The listing builds one solid part. Answer for the finished solid, in the listing's coordinates (mm). A direction names the side the tool comes from. Round coordinates to 2 decimals unless told otherwise and drop trailing zeros. Loops run counter-clockwise (first coordinate to the right, second up) from the corner with the lowest first, then second, coordinate; pieces in that order, holes last. Notation, with made-up numbers: M -40,8 L 12,8 A31 ccw 12,40 Z; hole C -24,10 d10. An arc over 180 degrees is marked long. Put each result on its own line as item: value. Start each with the question number.
(1) Which of the six approach directions +Z, -Z, +X, -X, +Y, -Y give full straight-line access (tool end or side, diameter ignored) to faces 4 (the face through (-17.02, -29.06, -7.32)), 5 (the face through (-23, 0, 0)), 6 (the face through (11.923, 3.755, 15.226))?
(2) Determine the mould class of faces 1 (the face through (-17.86, 17.92, -0.15)), 2 (the face through (20.48, -23.343, 0.175)), 3 (the face through (0, 0, 16.5)) for opening direction Z: released by +Z, released by -Z, zero draft, split by the parting line, or undercut.
(3) Section A-A, the plane z = 9 is taken. Determine the outline of the cut face in (x, y), then the cut area to 3 significant figures.
(4) Section D-D, the plane z = -6.5 is taken. Count the separate pieces of the cut face and the enclosed holes in it, then the cut area to 3 significant figures.
(5) Section C-C, the plane y = -27 is taken. Determine the outline of the cut face in (x, z).
(6) Straight lines are drawn through the part: line 1 (Y direction, x = 21, z = -4.25); line 2 (Y direction, x = -9.5, z = 9). For each, find the intervals that lie inside material, in ascending order.
(7) Flat-ended cylindrical pins translate along their axes: P1, Ø3, axis at x = -21, y = -21, coming from the +Z side; P2, Ø22, axis at x = 2.5, y = -2, coming from the +Z side; P3, Ø10.5, axis at x = -4, z = 3, coming from the -Y side; P4, Ø13, axis at x = 0, y = 0, coming from the +Z side. Find the tip coordinate at first contact, or state that the pin passes through.
```python
from build123d import *

# Parameters (mm, degrees)
SKETCH1_W            = 50
SKETCH1_H            = 50
BOSS_EXTRUDE1_DEPTH  = 12.5
SKETCH2_R            = 12.5
BOSS_EXTRUDE2_DEPTH  = 5
CUT_EXTRUDE1_REACH   = 45.301
SKETCH4_R            = 2.4
SKETCH5_R            = 13
BOSS_EXTRUDE3_DEPTH  = 1
SHELL1_START         = -10.5
SHELL1_DEPTH         = 21
SHELL1_START_2       = 10.5
SHELL1_2_OUTLINE_R   = 10.5
SHELL1_2_DEPTH       = 4
SHELL1_3_OUTLINE_R   = 11
SHELL1_3_OUTLINE_R_2 = 10.5
SHELL1_3_DEPTH       = 1
FILLET1_R            = 3
SKETCH6_R            = 10
CUT_EXTRUDE2_DEPTH   = 1
FILLET2_R            = 1
CHAMFER1_SIZE        = 0.5
SKETCH7_R            = 2.5
BOSS_EXTRUDE4_DEPTH  = 8
BOSS_EXTRUDE4_TAPER  = 5


# Read off the part's stored shape, not the designer's step: Shell1
with BuildPart() as part:
    # Sketch1 → Boss-Extrude1 (new, symmetric)
    with BuildSketch(Plane.XY):
        Rectangle(SKETCH1_W, SKETCH1_H)
    extrude(amount=BOSS_EXTRUDE1_DEPTH, both=True)

    # Sketch2 → Boss-Extrude2 (add)
    with BuildSketch(Plane.XY.offset(12.5)):
        Circle(SKETCH2_R)
    extrude(amount=BOSS_EXTRUDE2_DEPTH)

    # Sketch4 → Cut-Extrude1 (cut, up to next)
    with BuildSketch(Plane.XY.offset(12.5), mode=Mode.PRIVATE) as cut_extrude1_sk1:
        with Locations((-21, 21)):
            Circle(SKETCH4_R)
    cut_extrude1_tool1 = extrude(cut_extrude1_sk1.sketch, amount=-CUT_EXTRUDE1_REACH, mode=Mode.PRIVATE) & part.part
    # Sketch4 → Cut-Extrude1 (cut, up to next)
    with BuildSketch(Plane.XY.offset(12.5), mode=Mode.PRIVATE) as cut_extrude1_sk2:
        with Locations((21, 21)):
            Circle(SKETCH4_R)
    cut_extrude1_tool2 = extrude(cut_extrude1_sk2.sketch, amount=-CUT_EXTRUDE1_REACH, mode=Mode.PRIVATE) & part.part
    # Sketch4 → Cut-Extrude1 (cut, up to next)
    with BuildSketch(Plane.XY.offset(12.5), mode=Mode.PRIVATE) as cut_extrude1_sk3:
        with Locations((-21, -21)):
            Circle(SKETCH4_R)
    cut_extrude1_tool3 = extrude(cut_extrude1_sk3.sketch, amount=-CUT_EXTRUDE1_REACH, mode=Mode.PRIVATE) & part.part
    # Sketch4 → Cut-Extrude1 (cut, up to next)
    with BuildSketch(Plane.XY.offset(12.5), mode=Mode.PRIVATE) as cut_extrude1_sk4:
        with Locations((21, -21)):
            Circle(SKETCH4_R)
    cut_extrude1_tool4 = extrude(cut_extrude1_sk4.sketch, amount=-CUT_EXTRUDE1_REACH, mode=Mode.PRIVATE) & part.part
    add(cut_extrude1_tool1.solids().sort_by_distance((-21, 21, 12.5))[0], mode=Mode.SUBTRACT)
    add(cut_extrude1_tool2.solids().sort_by_distance((21, 21, 12.5))[0], mode=Mode.SUBTRACT)
    add(cut_extrude1_tool3.solids().sort_by_distance((-21, -21, 12.5))[0], mode=Mode.SUBTRACT)
    add(cut_extrude1_tool4.solids().sort_by_distance((21, -21, 12.5))[0], mode=Mode.SUBTRACT)

    # Sketch5 → Boss-Extrude3 (add)
    with BuildSketch(Plane.XY.offset(12.5)):
        Circle(SKETCH5_R)
    extrude(amount=BOSS_EXTRUDE3_DEPTH)

    # Shell1 outline → Shell1 (cut)
    with BuildSketch(Plane.XY.offset(SHELL1_START)):
        with BuildLine():
            Line((23, -17.080816412), (23, 17.080816412))
            ThreePointArc((23, 17.080816412), (17.888730163, 17.888730163), (17.080816412, 23))
            Line((17.080816412, 23), (-17.080816412, 23))
            ThreePointArc((-17.080816412, 23), (-17.888730163, 17.888730163), (-23, 17.080816412))
            Line((-23, 17.080816412), (-23, -17.080816412))
            ThreePointArc((-23, -17.080816412), (-17.888730163, -17.888730163), (-17.080816412, -23))
            Line((-17.080816412, -23), (17.080816412, -23))
            ThreePointArc((17.080816412, -23), (17.888730163, -17.888730163), (23, -17.080816412))
        make_face()
    extrude(amount=SHELL1_DEPTH, mode=Mode.SUBTRACT)

    # Shell1 2 outline → Shell1 2 (cut)
    with BuildSketch(Plane.XY.offset(SHELL1_START_2)):
        Circle(SHELL1_2_OUTLINE_R)
    extrude(amount=SHELL1_2_DEPTH, mode=Mode.SUBTRACT)

    # Shell1 3 outline → Shell1 3 (cut)
    with BuildSketch(Plane.XY.offset(SHELL1_START_2)):
        Circle(SHELL1_3_OUTLINE_R)
        Circle(SHELL1_3_OUTLINE_R_2, mode=Mode.SUBTRACT)
    extrude(amount=SHELL1_3_DEPTH, mode=Mode.SUBTRACT)

    # Fillet1
    fillet1_edges = [part.edges().sort_by_distance(p)[0] for p in [
        (23, 17.080816412, 0),
        (-17.080816412, 23, 0),
        (-23, -17.080816412, 0),
        (17.080816412, -23, 0),
        (-23, 17.080816412, 0),
        (-17.080816412, -23, 0),
        (17.080816412, 23, 0),
    ]]
    fillet(fillet1_edges, radius=FILLET1_R)

    # Sketch6 → Cut-Extrude2 (cut)
    with BuildSketch(Plane.XY.offset(17.5)):
        Circle(SKETCH6_R)
    extrude(amount=-CUT_EXTRUDE2_DEPTH, mode=Mode.SUBTRACT)

    # Fillet2
    # the kernel refuses this fillet: 1 mm, written as the material it takes off along each edge
    with BuildSketch(Plane(origin=(0, 0, 13.5), x_dir=(1, 0, 0), z_dir=(0, -1, 0))) as fillet2_piece_1:
        with BuildLine():
            CenterArc((12, -0.866025404), FILLET2_R, 0, 60)
            Line((12.5, 0), (12.51, 0.017320508))
            ThreePointArc((12.51, 0.017320508), (12.75, 0.02), (13, 0.02))
            Line((13, 0.02), (13.02, 0))
            Line((13.02, 0), (13.02, -0.866025404))
            Line((13.02, -0.866025404), (13, -0.866025404))
        make_face()
    revolve(axis=Axis((0, 0, 13.5), (0, 0, 1)), mode=Mode.SUBTRACT)

    # Chamfer1
    chamfer1_edges = [part.edges().sort_by_distance(p)[0] for p in [
        (-12.5, 0, 17.5),
    ]]
    chamfer(chamfer1_edges, length=CHAMFER1_SIZE)

    # Sketch7 → Boss-Extrude4 (add)
    with BuildSketch(Plane.XZ.offset(25)):
        with Locations((-19, -6.5)):
            Circle(SKETCH7_R)
    extrude(amount=BOSS_EXTRUDE4_DEPTH, taper=BOSS_EXTRUDE4_TAPER)


solid = part.part
```
Recorded:
1. face 4: -Y
1. face 5: none
1. face 6: +Z
2. face 1: undercut
2. face 2: zero draft
2. face 3: released by +Z
3. outline: M -25,-25 L 25,-25 L 25,25 L -25,25 Z; hole C -21,-21 d4.8; hole C -21,21 d4.8; hole M -23,-13.67 A3 ccw -20.41,-16.64 A4.4 cw -16.64,-20.41 A3 ccw -13.67,-23 L 13.67,-23 A3 ccw 16.64,-20.41 A4.4 cw 23,-17.08 L 23,13.67 A3 ccw 20.41,16.64 A4.4 cw 16.64,20.41 A3 ccw 13.67,23 L -13.67,23 A3 ccw -16.64,20.41 A4.4 cw -20.41,16.64 A3 ccw -23,13.67 Z; hole C 21,-21 d4.8; hole C 21,21 d4.8
3. area: 471 mm²
4. separate pieces: 1
4. enclosed holes: 5
4. area: 505 mm²
5. outline: C -19,-6.5 d4.65
6. line 1: y = -25 to -23.4, -18.6 to -16.6, 16.5 to 18.6, 23.4 to 25
6. line 2: y = -25 to -23, 23 to 25
7. P1: passes through
7. P2: stops at z = 17.5
7. P3: stops at y = -25
7. P4: stops at z = 16.5
